The model under review builds one solid part; all positions refer to its coordinate system, in mm. Give positions to 0.01 mm unless a question says otherwise; leave off trailing zeros. Loops run counter-clockwise (first coordinate to the right, second up) from the corner with the lowest first, then second, coordinate; pieces in that order, holes last. Notation, with made-up numbers: M 21,-33 L 56,-33 A16 ccw 56,-12 Z; hole C -18,19.5 d11. An arc over 180 degrees is marked long. One line per item, written item: value. Start each with the question number.
Q1. For pin 1 (6 mm diameter, centred on x = -2.5, z = 709, fed in from +Y); pin 2 (6 mm diameter, centred on x = 4, z = 216.5, fed in from -Y); pin 3 (8 mm diameter, centred on y = -4, z = 719, fed in from +X), all flat-tipped, find the tip position at first contact; note any pin that passes through.
Q2. To check wall thickness, follow line 1 along Y through (x, z) = (3.25, 431.5); line 2 along X through (y, z) = (1.75, 206); line 3 along X through (y, z) = (1, 415). State the ranges of each line that lie inside material, in increasing order. Write a range as from..to.
Q3. We need section A-A on z = 693.5. Write out the cut boundary in (x, y), plus the area to 3 significant figures.
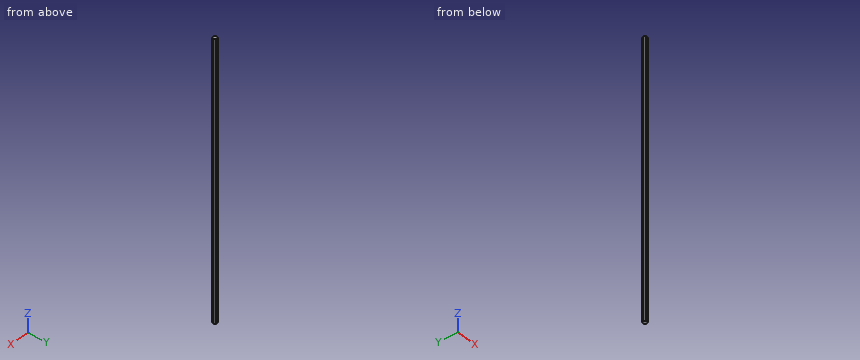
Autodesk Inventor part; units mm, degrees
ref_plane "YZ Plane" through (0, 0, 0) normal (1, 0, 0) x (0, 1, 0)
ref_plane "XZ Plane" through (0, 0, 0) normal (0, 1, 0) x (-1, 0, 0)
ref_plane "XY Plane" through (0, 0, 0) normal (0, 0, 1) x (1, 0, 0)
sketch "Sketch1" plane through (0, 0, 0) normal (0, 0, 1) x (1, 0, 0)
  arc A0 (-5.109, 4.6004) -> (-6.8651, -0.3684) centre (0, 0) ccw
  line L0 (-4.7654, 5.5726) -> (-3.7516, 5.7612)
  line L1 (2.4434, 6.9133) -> (3.1135, 6.1296)
  line L2 (7.2087, 1.3406) -> (6.8651, 0.3684)
  line L3 (4.7654, -5.5726) -> (3.7516, -5.7612)
  line L4 (-2.4434, -6.9133) -> (-3.1135, -6.1296)
  line L5 (-7.2087, -1.3406) -> (-6.8651, -0.3684)
  arc A1 (-3.7516, 5.7612) -> (-5.109, 4.6004) centre (0, 0) ccw
  arc A2 (1.4295, 6.7247) -> (-3.7516, 5.7612) centre (0, 0) ccw
  arc A3 (3.1135, 6.1296) -> (1.4295, 6.7247) centre (0, 0) ccw
  arc A4 (6.5386, 2.1243) -> (3.1135, 6.1296) centre (0, 0) ccw
  arc A5 (6.8651, 0.3684) -> (6.5386, 2.1243) centre (0, 0) ccw
  arc A6 (5.109, -4.6004) -> (6.8651, 0.3684) centre (0, 0) ccw
  arc A7 (3.7516, -5.7612) -> (5.109, -4.6004) centre (0, 0) ccw
  arc A8 (-1.4295, -6.7247) -> (3.7516, -5.7612) centre (0, 0) ccw
  arc A9 (-3.1135, -6.1296) -> (-1.4295, -6.7247) centre (0, 0) ccw
  arc A10 (-6.5386, -2.1243) -> (-3.1135, -6.1296) centre (0, 0) ccw
  arc A11 (-6.8651, -0.3684) -> (-6.5386, -2.1243) centre (0, 0) ccw
  line L6 (-5.109, 4.6004) -> (-4.7654, 5.5726)
  line L7 (-6.8651, -0.3684) -> (-5.109, 4.6004)
  line L8 (-6.5386, -2.1243) -> (-7.2087, -1.3406)
  line L9 (-3.1135, -6.1296) -> (-6.5386, -2.1243)
  line L10 (-1.4295, -6.7247) -> (-2.4434, -6.9133)
  line L11 (3.7516, -5.7612) -> (-1.4295, -6.7247)
  line L12 (5.109, -4.6004) -> (4.7654, -5.5726)
  line L13 (6.8651, 0.3684) -> (5.109, -4.6004)
  line L14 (6.5386, 2.1243) -> (7.2087, 1.3406)
  line L15 (3.1135, 6.1296) -> (6.5386, 2.1243)
  line L16 (1.4295, 6.7247) -> (2.4434, 6.9133)
  line L17 (-3.7516, 5.7612) -> (1.4295, 6.7247)
  dimension "d0" = 12.7
  dimension "d1" = 13.75
extrude "Extrusion1" add sketch "Sketch1" along normal blind 914.4 contours A1 L17 A3 L15 A5 L13 A7 L11 A9 L9 A11 L7
properties part number "ThunderHex36"
Solved:
1. pin 1: y = 6.55
1. pin 2: y = -6.27
1. pin 3: x = 6.73
2. line 1: -5.85..5.97
2. line 2: -6.12..6.65
2. line 3: -6.38..6.8
3. outline: M -6.87,-0.37 A6.88 ccw -6.54,-2.12 L -3.11,-6.13 A6.87 ccw -1.43,-6.72 L 3.75,-5.76 A6.87 ccw 5.11,-4.6 L 6.87,0.37 A6.88 ccw 6.54,2.12 L 3.11,6.13 A6.87 ccw 1.43,6.72 L -3.75,5.76 A6.87 ccw -5.11,4.6 Z
3. area: 137 mm2
